Verification items for the finished model (mm, model axes). A direction names the side the tool comes from. Coordinates: 2 decimals unless noted, no trailing zeros. Loops run counter-clockwise (first coordinate to the right, second up) from the corner with the lowest first, then second, coordinate; pieces in that order, holes last. Notation, with made-up numbers: (0.5, -4) -> (40.5, -4) arc R23 cw to (40.5, 9) -> close; hole circle Ø9 at (59.25, 4.5). An arc over 180 degrees is marked (long way). Use CSV: the item, a comma, the result in double quotes. Start each with the question number.
```python
from build123d import *

# Parameters (mm, degrees)
SKETCH_1_R               = 10
SKETCH_1_R_2             = 7.5
EXTRUDE_1_DEPTH          = 250
EXTRUDE_2_DEPTH          = 5
EXTRUDE_2_DEPTH_BACK     = 10
CUT_EXTRUDE_1_DEPTH      = 252.25286068
CUT_EXTRUDE_1_DEPTH_BACK = 252.25286068
FILLET_1_R               = 1
SKETCH_5_R               = 4
SKETCH_5_R_2             = 2
CUT_EXTRUDE_2_DEPTH      = 5


with BuildPart() as part:
    # 草图1 → 凸台-拉伸1 (new body)
    with BuildSketch(Plane(origin=(0, 0, 0), x_dir=(1, 0, 0), z_dir=(0, 1, 0))):
        with Locations(Location((0, 0, 0), (0, 0, 270))):
            Circle(SKETCH_1_R)
        with Locations(Location((0, 0, 0), (0, 0, 270))):
            Circle(SKETCH_1_R_2, mode=Mode.SUBTRACT)
    extrude(amount=EXTRUDE_1_DEPTH)

    # 草图2 → 凸台-拉伸2 (add, two sides: drawn at the far end of the back side and taken through both)
    with BuildSketch(Plane(origin=(0, 0, 0), x_dir=(1, 0, 0), z_dir=(0, 1, 0)).offset(-EXTRUDE_2_DEPTH_BACK)):
        with BuildLine():
            Line((10, -12), (-2, -12))
            ThreePointArc((-2, -12), (-14, 0), (-2, 12))
            Line((-2, 12), (10, 12))
            ThreePointArc((10, 12), (22, 0), (10, -12))
        make_face()
    extrude(amount=EXTRUDE_2_DEPTH + EXTRUDE_2_DEPTH_BACK)

    # 草图4 → 切除-拉伸1 (cut, two sides: drawn at the far end of the back side and taken through both)
    with BuildSketch(Plane.XY.offset(-CUT_EXTRUDE_1_DEPTH_BACK)):
        Polygon((-14, -1.688745119), (-14, -10), (22, -10), align=None)
    extrude(amount=CUT_EXTRUDE_1_DEPTH + CUT_EXTRUDE_1_DEPTH_BACK, mode=Mode.SUBTRACT)

    # 圆角1
    fillet_1_edges = [part.edges().sort_by_distance(p)[0] for p in [
        (0, 5, -10),
        (22, 5, 0),
        (4, 5, -12),
        (-14, 5, 0),
        (4, 5, 12),
        (18.485281374, -9.188563269, -8.485281374),
        (-10.485281374, -2.500181851, 8.485281374),
        (4, -5.84437256, 12),
        (4, -5.84437256, -12),
    ]]
    fillet(fillet_1_edges, radius=FILLET_1_R - 0.0001)  # a hair under: the kernel refuses the full size

    # 草图5 → 切除-拉伸2 (cut)
    with BuildSketch(Plane(origin=(-1.078590243, -4.671887617, 0), x_dir=(0.9743700647852368, -0.22495105434385856, 0), z_dir=(-0.22495105434385856, -0.9743700647852368, 0))):
        with Locations((-5, 0)):
            Circle(SKETCH_5_R)
        with Locations((5.392304845, 6)):
            Circle(SKETCH_5_R_2)
        with Locations((5.392304845, -6)):
            Circle(SKETCH_5_R_2)
    extrude(amount=-CUT_EXTRUDE_2_DEPTH, mode=Mode.SUBTRACT)


solid = part.part
```
1. Set-up check for faces 5 (the cylindrical face through (-6.241, -0.95, -3.905)), 6 (the flat face through (12, 5, 1)): record each of +Z, -Z, +X, -X, +Y, -Y from which the full face is reachable in a straight line by a thin tool's end or side.
2. Release check for a two-part mould opening along X. For faces 1 (the cylindrical face through (22, -2, 0)), 2 (the flat face through (7, 250, 4)), 3 (the cylindrical face through (-9.76, 126.29, -2.17)), 4 (the flat face through (-4.88, 1.337, 0.056)) record: released by +X, released by -X, zero draft, split by the parting line, or undercut.
3. Scan lines: line 1 (Z direction, x = 0, y = 158.5); line 2 (X direction, y = 57, z = 3.25). Record each from-to range of solid material in increasing order.
4. Cross-section at A-A, the plane y = 213. Record the boundary of the cut face in (x, z), plus the area to 3 significant figures.
5. Depth check by flat-ended pin: pin 1 (10 mm diameter, centred on x = -2, y = 109.5, fed in from -Z); pin 2 (6 mm diameter, centred on x = -4, y = 182.5, fed in from -Z); pin 3 (6 mm diameter, centred on x = 4.5, y = 34, fed in from +Z). Enter the tip coordinate at first touch or a pass-through.
Solution:
1,face 5,"none"
1,face 6,"+Y"
2,face 1,"released by +X"
2,face 2,"zero draft"
2,face 3,"split by the parting line"
2,face 4,"undercut"
3,line 1,"z = -10 to -7.5, 7.5 to 10"
3,line 2,"x = -9.46 to -6.76, 6.76 to 9.46"
4,outline,"circle Ø20 at (0, 0); hole circle Ø15 at (0, 0)"
4,area,"137 mm2"
5,pin 1,"stops at z = -10"
5,pin 2,"stops at z = -9.95"
5,pin 3,"stops at z = 9.89"
